Autodesk Inventor part; units mm, degrees
ref_plane "YZ Plane" through (0, 0, 0) normal (1, 0, 0) x (0, 1, 0)
ref_plane "XZ Plane" through (0, 0, 0) normal (0, 1, 0) x (-1, 0, 0)
ref_plane "XY Plane" through (0, 0, 0) normal (0, 0, 1) x (1, 0, 0)
sketch "Sketch1" plane through (0, 0, 0) normal (0, 1, 0) x (-1, 0, 0)
  line L0 (0, 0) -> (685.8, 0)
  line L1 (685.8, 0) -> (685.8, -304.8)
  line L2 (685.8, -304.8) -> (0, -304.8)
  line L3 (0, -304.8) -> (0, 0)
  line L4 (685.8, 0) -> (0, 0)
  line L5 (0, 0) -> (0, 120.65)
  line L6 (0, 120.65) -> (685.8, 120.65)
  line L7 (685.8, 120.65) -> (685.8, 0)
  dimension "d0" = 685.8
  dimension "d1" = 304.8
  dimension "d4" = 120.65
extrude "Extrusion1" add sketch "Sketch1" along normal blind 5.08 contours L0 L1 L2 L3
sketch "Sketch2" plane through (-685.8, 0, 0) normal (0, 0, 1) x (1, 0, 0)
  line L0 (685.8, 0) -> (0, 0)
  line L1 (685.8, 0) -> (685.8, 5.08)
  line L2 (0, 5.08) -> (685.8, 5.08)
  line L3 (0, 0) -> (0, 5.08)
extrude "Extrusion2" add sketch "Sketch2" along normal blind 120.65
sketch "Sketch3" plane through (0, 5.08, 0) normal (0, 1, 0) x (1, 0, 0)
  point P0 (0, 0)
sketch "Sketch4" plane through (0, 5.08, 0) normal (0, 1, 0) x (1, 0, 0)
  line L0 (-685.8, -120.65) -> (-685.8, 304.8)
  line L1 (-685.8, 92.075) -> (-609.6, 92.075)
  line L2 (-609.6, 92.075) -> (-609.6, -34.925)
  line L3 (-609.6, 92.075) -> (-609.6, 219.075)
  line L4 (-609.6, 219.075) -> (-406.4, 219.075)
  line L5 (-406.4, 219.075) -> (-406.4, -34.925)
  line L6 (-406.4, -34.925) -> (-609.6, -34.925)
  line L7 (0, 304.8) -> (0, -120.65)
  line L8 (0, 92.075) -> (-69.85, 92.075)
  line L9 (-69.85, 92.075) -> (-69.85, 219.075)
  line L10 (-69.85, 219.075) -> (-273.05, 219.075)
  line L11 (-273.05, 219.075) -> (-273.05, -34.925)
  line L12 (-273.05, -34.925) -> (-69.85, -34.925)
  line L13 (-69.85, -34.925) -> (-69.85, 92.075)
  line L14 (-419.1, -22.225) -> (-419.1, 206.375)
  line L15 (-419.1, 206.375) -> (-596.9, 206.375)
  line L16 (-596.9, 206.375) -> (-596.9, 92.075)
  line L17 (-596.9, 92.075) -> (-596.9, -22.225)
  line L18 (-596.9, -22.225) -> (-419.1, -22.225)
  line L19 (-260.35, -22.225) -> (-260.35, 206.375)
  line L20 (-260.35, 206.375) -> (-82.55, 206.375)
  line L21 (-82.55, 206.375) -> (-82.55, 92.075)
  line L22 (-82.55, 92.075) -> (-82.55, -22.225)
  line L23 (-82.55, -22.225) -> (-260.35, -22.225)
  point P0 (0, 0)
  dimension "d7" = 76.2
  dimension "d8" = 127
  dimension "d9" = 127
  dimension "d10" = 203.2
  dimension "d11" = 69.85
  dimension "d12" = 203.2
  dimension "d13" = 12.7
  dimension "d14" = 12.7
extrude "Extrusion3" cut sketch "Sketch4" against normal blind 25.4 contours L18 L17 L16 L15 L14 | L19 L20 L21 L22 L23
sketch "Sketch5" plane through (0, 5.08, 0) normal (0, 1, 0) x (1, 0, 0)
  point P0 (0, 0)
sketch "Sketch6" plane through (0, 5.08, 0) normal (0, 1, 0) x (1, 0, 0)
  line L0 (-596.9, 206.375) -> (-419.1, 206.375)
  line L1 (-419.1, 206.375) -> (-419.1, -22.225)
  line L2 (-419.1, -22.225) -> (-596.9, -22.225)
  line L3 (-596.9, -22.225) -> (-596.9, 206.375)
  line L4 (-82.55, -22.225) -> (-260.35, -22.225)
  line L5 (-260.35, -22.225) -> (-260.35, 206.375)
  line L6 (-260.35, 206.375) -> (-82.55, 206.375)
  line L7 (-82.55, 206.375) -> (-82.55, -22.225)
  line L8 (0, 304.8) -> (0, -120.65)
  line L9 (0, 304.8) -> (-685.8, 304.8)
  line L10 (-685.8, 304.8) -> (-685.8, -120.65)
  line L11 (0, -120.65) -> (-685.8, -120.65)
  line L12 (-596.9, 206.375) -> (-419.1, 206.375)
  line L13 (-419.1, 206.375) -> (-419.1, -22.225)
  line L14 (-419.1, -22.225) -> (-596.9, -22.225)
  line L15 (-596.9, -22.225) -> (-596.9, 206.375)
  line L16 (-419.1, 206.375) -> (-419.1, -22.225)
  line L17 (-260.35, 206.375) -> (-82.55, 206.375)
  line L18 (-82.55, 206.375) -> (-82.55, -22.225)
  line L19 (-82.55, -22.225) -> (-260.35, -22.225)
  line L20 (-260.35, -22.225) -> (-260.35, 206.375)
  line L21 (-508, -22.225) -> (-508, 206.375)
  line L22 (-596.9, -22.225) -> (-596.9, 206.375)
  line L23 (-596.9, 92.075) -> (-419.1, 92.075)
  line L24 (-171.45, 206.375) -> (-171.45, -22.225)
  line L25 (-82.55, 92.075) -> (-260.35, 92.075)
  point P0 (0, 0)
  point P1 (-508, 92.075)
  point P2 (-171.45, 92.075)
sketch "Sketch7" plane through (0, 5.08, 0) normal (0, 1, 0) x (1, 0, 0)
  line L0 (-596.9, 206.375) -> (-419.1, 206.375)
  line L1 (-419.1, 206.375) -> (-419.1, -22.225)
  line L2 (-419.1, -22.225) -> (-596.9, -22.225)
  line L3 (-596.9, -22.225) -> (-596.9, 206.375)
  line L4 (-82.55, -22.225) -> (-260.35, -22.225)
  line L5 (-260.35, -22.225) -> (-260.35, 206.375)
  line L6 (-260.35, 206.375) -> (-82.55, 206.375)
  line L7 (-82.55, 206.375) -> (-82.55, -22.225)
  line L8 (0, 304.8) -> (0, -120.65)
  line L9 (0, 304.8) -> (-685.8, 304.8)
  line L10 (-685.8, 304.8) -> (-685.8, -120.65)
  line L11 (0, -120.65) -> (-685.8, -120.65)
  line L12 (-381, 34.925) -> (-304.8, 34.925)
  line L13 (-304.8, 34.925) -> (-304.8, 149.225)
  line L14 (-304.8, 149.225) -> (-381, 149.225)
  line L15 (-381, 149.225) -> (-381, 34.925)
  line L16 (-381, 34.925) -> (-304.8, 149.225) construction
  line L17 (-304.8, 34.925) -> (-381, 149.225) construction
  point P0 (0, 0)
  point P1 (-342.9, 92.075)
  dimension "d17" = 76.2
  dimension "d18" = 114.3
extrude "Extrusion4" cut sketch "Sketch7" against normal blind 25.4 contours L15 L14 L13 L12
properties part number "cart_woodpanel-front" material "Wood (Birch)"
Could you check a few things on this model? Use its own coordinates, in mm. Coordinates: 2 decimals unless noted, no trailing zeros. Loops run counter-clockwise (first coordinate to the right, second up) from the corner with the lowest first, then second, coordinate; pieces in that order, holes last. Notation, with made-up numbers: M -6,-25.75 L 10,-25.75 A17 cw 10,-13.75 Z; hole C 63.25,16 d3. An arc over 180 degrees is marked long. Put each result on its own line as item: value. Start each with the question number.
(1) Suppose I cut it at C-C on y = 2.6. Please give me the cut outline in (x, z) (3 decimals), then the cut area to 3 significant figures.
(2) I need wall thicknesses on line 1 (X direction, y = 1.6, z = -178); line 2 (X direction, y = 0.85, z = -68.5); line 3 (Z direction, x = -166.5, y = 1.4) (3 decimals). Which ranges of each line are inside material? Lowest first, please. Write a range as from..to.
(3) Suppose I cut it at D-D on z = -134.5. Please give me the cut outline in (x, y), then the cut area to 3 significant figures.
(4) Suppose I cut it at B-B on z = 3. Please give me the cut outline in (x, y).
(5) Thinking about a two-plate mould opening in Y: for faces 1 (the face through (-262, 5.08, -89)), 2 (the face through (-262, 0, -89)), which applies, pulls with the +Y half, pulls with the -Y half, needs draft (parallel to the pull), parting line crosses it, or undercut?
(6) Suppose I cut it at A-A on x = -347. Please give me the cut outline in (y, z) (3 decimals), then the cut area to 3 significant figures.
Solutions:
1. outline: M -685.8,-304.8 L 0,-304.8 L 0,120.65 L -685.8,120.65 Z; hole M -596.9,-206.375 L -419.1,-206.375 L -419.1,22.225 L -596.9,22.225 Z; hole M -381,-149.225 L -304.8,-149.225 L -304.8,-34.925 L -381,-34.925 Z; hole M -260.35,-206.375 L -82.55,-206.375 L -82.55,22.225 L -260.35,22.225 Z
1. area: 202,000 mm2
2. line 1: x = -685.8..-596.9, -419.1..-260.35, -82.55..0
2. line 2: x = -685.8..-596.9, -419.1..-381, -304.8..-260.35, -82.55..0
2. line 3: z = -304.8..-206.375, 22.225..120.65
3. outline: M -685.8,0 L -596.9,0 L -596.9,5.08 L -685.8,5.08 Z; M -419.1,0 L -381,0 L -381,5.08 L -419.1,5.08 Z; M -304.8,0 L -260.35,0 L -260.35,5.08 L -304.8,5.08 Z; M -82.55,0 L 0,0 L 0,5.08 L -82.55,5.08 Z
3. area: 1,290 mm2
4. outline: M -685.8,0 L -596.9,0 L -596.9,5.08 L -685.8,5.08 Z; M -419.1,0 L -260.35,0 L -260.35,5.08 L -419.1,5.08 Z; M -82.55,0 L 0,0 L 0,5.08 L -82.55,5.08 Z
5. face 1: pulls with the +Y half
5. face 2: pulls with the -Y half
6. outline: M 0,-304.8 L 5.08,-304.8 L 5.08,-149.225 L 0,-149.225 Z; M 0,-34.925 L 5.08,-34.925 L 5.08,120.65 L 0,120.65 Z
6. area: 1,580 mm2
